Build history of the part. All positions in model axes, mm. A direction names the side the tool comes from. Round coordinates to 2 decimals unless told otherwise and drop trailing zeros. Write each loop counter-clockwise with the first axis right and the second up, starting at its lowest first coordinate (ties: lowest second). Pieces come first, ordered by that corner, then holes. Notation, with made-up numbers: M 71.5,-10.75 L 87.5,-10.75 A8 ccw 87.5,-0.75 Z; hole C 89.25,25.25 d9. An arc over 180 degrees is marked long. Write item = value, one per line.
from build123d import *

# Parameters (mm, degrees)
ESQUISSE1_W             = 151
ESQUISSE1_H             = 65
BOSS_EXTRU_1_DEPTH      = 77.5
ESQUISSE3_W             = 148.454907539
ESQUISSE3_H             = 62.58067557
BOSS_EXTRU_4_DEPTH      = 1
ESQUISSE4_W             = 151
ESQUISSE4_H             = 65
BOSS_EXTRU_5_DEPTH      = 19
ESQUISSE5_W             = 5.004872729
ESQUISSE5_H             = 5.013872644
ESQUISSE5_H_2           = 5.00047463
ENL_V_MAT_EXTRU_1_DEPTH = 159
ESQUISSE6_W             = 15.091858935
ESQUISSE6_H             = 6.446271405
BOSS_EXTRU_6_DEPTH      = 5
ESQUISSE7_W             = 13.28107707
ESQUISSE7_H             = 3.860939677
ENL_V_MAT_EXTRU_2_DEPTH = 45
ESQUISSE8_W             = 1.776428529
ESQUISSE8_H             = 6.399764331
BOSS_EXTRU_7_DEPTH      = 0.25


with BuildPart() as part:
    # Esquisse1 → Boss.-Extru.1 (new body)
    with BuildSketch(Plane.XY):
        with Locations((75.5, 32.5)):
            Rectangle(ESQUISSE1_W, ESQUISSE1_H)
    extrude(amount=BOSS_EXTRU_1_DEPTH)

    # Esquisse3 → Boss.-Extru.4 (add)
    with BuildSketch(Plane.XY.offset(77.5)):
        with Locations((75.821779061, 32.317365634)):
            Rectangle(ESQUISSE3_W, ESQUISSE3_H)
    extrude(amount=BOSS_EXTRU_4_DEPTH)

    # Esquisse4 → Boss.-Extru.5 (add)
    with BuildSketch(Plane.XY.offset(78.5)):
        with Locations((75.5, 32.5)):
            Rectangle(ESQUISSE4_W, ESQUISSE4_H)
    extrude(amount=BOSS_EXTRU_5_DEPTH)

    # Esquisse5 → Enlèv. mat.-Extru.1 (cut)
    with BuildSketch(Plane(origin=(151, 0, 0), x_dir=(0, 0, -1), z_dir=(1, 0, 0))):
        with Locations((-94.997563636, 2.506936322)):
            Rectangle(ESQUISSE5_W, ESQUISSE5_H)
        with Locations((-94.997563636, 62.499762685)):
            Rectangle(ESQUISSE5_W, ESQUISSE5_H_2)
    extrude(amount=-ENL_V_MAT_EXTRU_1_DEPTH, mode=Mode.SUBTRACT)

    # Esquisse6 → Boss.-Extru.6 (add)
    with BuildSketch(Plane.XY.offset(97.5)):
        with Locations((138.863055981, 49.690815345)):
            Rectangle(ESQUISSE6_W, ESQUISSE6_H)
        with Locations((138.863055981, 15.32258267)):
            Rectangle(ESQUISSE6_W, ESQUISSE6_H)
    extrude(amount=BOSS_EXTRU_6_DEPTH)

    # Esquisse7 → Enlèv. mat.-Extru.2 (cut)
    with BuildSketch(Plane(origin=(0, 52.913951047, 0), x_dir=(1, 0, 0), z_dir=(0, 1, 0))):
        with Locations((137.957665049, -99.430469839)):
            Rectangle(ESQUISSE7_W, ESQUISSE7_H)
    extrude(amount=-ENL_V_MAT_EXTRU_2_DEPTH, mode=Mode.SUBTRACT)

    # Esquisse8 → Boss.-Extru.7 (add)
    with BuildSketch(Plane.XY.offset(97.5)):
        with Locations((147.886510026, 15.299329133)):
            Rectangle(ESQUISSE8_W, ESQUISSE8_H)
    extrude(amount=BOSS_EXTRU_7_DEPTH)


solid = part.part
1. Band-saw the part on A-A (y = 22). List the corners of the cut face in (x, z), plus the area to 3 significant figures.
Responses:
outline = M 0,0 L 151,0 L 151,77.5 L 150.05,77.5 L 150.05,78.5 L 151,78.5 L 151,97.5 L 0,97.5 L 0,78.5 L 1.59,78.5 L 1.59,77.5 L 0,77.5 Z
area = 14,700 mm²
2. Band-saw the part on C-C (y = 51). List the corners of the cut face in (x, z).
Responses:
outline = M 0,0 L 151,0 L 151,77.5 L 150.05,77.5 L 150.05,78.5 L 151,78.5 L 151,97.5 L 146.41,97.5 L 146.41,102.5 L 131.32,102.5 L 131.32,101.36 L 144.6,101.36 L 144.6,97.5 L 0,97.5 L 0,78.5 L 1.59,78.5 L 1.59,77.5 L 0,77.5 Z
3. Probe probe 1 along Z at (x, y) = (44, 33.5); probe 2 along Y at (x, z) = (53, 96). List the from-to ranges inside material, lowest first.
Responses:
probe_1 = 0 to 97.5
probe_2 = 5.01 to 60
4. Band-saw the part on B-B (x = 85). List the corners of the cut face in (y, z).
Responses:
outline = M 0,0 L 65,0 L 65,77.5 L 63.61,77.5 L 63.61,78.5 L 65,78.5 L 65,92.5 L 60,92.5 L 60,97.5 L 5.01,97.5 L 5.01,92.5 L 0,92.5 L 0,78.5 L 1.03,78.5 L 1.03,77.5 L 0,77.5 Z
5. Flat gauge pins, fed straight in: pin 1 (2.5 mm diameter, centred on x = 63.5, z = 95.5, fed in from -Y); pin 2 (1.9 mm diameter, centred on y = 15, z = 100, fed in from -X); pin 3 (4 mm diameter, centred on y = 48, z = 100, fed in from +X). Where does each tip first touch, or does it go through?
Responses:
pin_1 = 5.01
pin_2 = 144.6
pin_3 = 146.41
6. Tool access for faces 1 (the face through (77, 5.014, 95)), 2 (the face through (146.409, 50, 100)), 3 (the face through (141, 18.546, 102)): list every direction of +Z, -Z, +X, -X, +Y, -Y with a clear straight run to the whole face (end or side of a thin tool).
Responses:
face_1 = +Z, +X, -X, -Y
face_2 = +Z, +X, +Y, -Y
face_3 = +Z, +X, -X
7. Mould opens along Z. For faces 4 (the face through (139, 50, 102.5)), 5 (the face through (75, 64, 78.5)), 6 (the face through (77, 60, 95)) say: pulls with the +Z half, pulls with the -Z half, needs draft (parallel to the pull), parting line crosses it, or undercut.
Responses:
face_4 = pulls with the +Z half
face_5 = undercut
face_6 = needs draft
